from build123d import *

# Parameters (mm, degrees)
SKETCH1_R                = 57.15
SKETCH1_R_2              = 51.1302
SCHEDULED_CHAMBER_DEPTH  = 260.35
SKETCH2_R                = 76.2
SKETCH2_R_2              = 54.102
FLANGE_DEPTH             = 6.35
ORIGINAL_BOLT_HOLE_REACH = 283.771
SKETCH3_R                = 3.175
BOLT_HOLE_PATTERN_COUNT  = 8


with BuildPart() as part:
    # Sketch1 → Scheduled Chamber (new body)
    with BuildSketch(Plane(origin=(0, 0, 0), x_dir=(1, 0, 0), z_dir=(0, 1, 0))):
        with Locations(Location((0, 0, 0), (0, 0, 270))):
            Circle(SKETCH1_R)
        with Locations(Location((0, 0, 0), (0, 0, 270))):
            Circle(SKETCH1_R_2, mode=Mode.SUBTRACT)
    extrude(amount=-SCHEDULED_CHAMBER_DEPTH)

    # Sketch2 → Flange (add)
    with BuildSketch(Plane(origin=(0, 0, 0), x_dir=(1, 0, 0), z_dir=(0, 1, 0))):
        with Locations(Location((0, 0, 0), (0, 0, 270))):
            Circle(SKETCH2_R)
        Circle(SKETCH2_R_2, mode=Mode.SUBTRACT)
    extrude(amount=-FLANGE_DEPTH)

    # Sketch3 → Original Bolt Hole (cut, up to next)
    with BuildSketch(Plane(origin=(0, 0, 0), x_dir=(1, 0, 0), z_dir=(0, 1, 0)), mode=Mode.PRIVATE) as original_bolt_hole_sk1:
        with Locations(Location((0, 68.58, 0), (0, 0, 270))):
            Circle(SKETCH3_R)
    original_bolt_hole_tool1 = extrude(original_bolt_hole_sk1.sketch, amount=-ORIGINAL_BOLT_HOLE_REACH, mode=Mode.PRIVATE) & part.part
    original_bolt_hole = original_bolt_hole_tool1.solids().sort_by_distance((0, 0, -68.58))[0]
    add(original_bolt_hole, mode=Mode.SUBTRACT)

    # Bolt Hole Pattern: Original Bolt Hole ×8 about axis
    bolt_hole_pattern_axis = Axis((0, 0, 0), (0, 1, 0))
    for i in range(1, BOLT_HOLE_PATTERN_COUNT):
        add(original_bolt_hole.rotate(bolt_hole_pattern_axis, i * 360 / BOLT_HOLE_PATTERN_COUNT), mode=Mode.SUBTRACT)


solid = part.part
Can you work these out from the model? Positions are in its coordinate system, mm. A direction names the side the tool comes from. Give positions to 0.01 mm unless a question says otherwise; leave off trailing zeros. Order: outer loops, then holes, each group sorted by start corner. A loop starts at its lowest first (then second) coordinate and runs counter-clockwise, first axis right, second up. Notation, with made-up numbers: (30, -37.5) - (63, -37.5) arc R19 ccw to (63, -30.5) - close; hole circle Ø10 at (29, 66.25). An arc over 180 degrees is marked (long way). Write each question's results on one line, items separated by ' | '.
1) Suppose I cut it at C-C, the plane x = -16. Write out the boundary of the cut face in (y, z).
Final values:
outline: (-260.35, -54.86) - (-6.35, -54.86) - (-6.35, -74.5) - (0, -74.5) - (0, -48.56) - (-260.35, -48.56) - close; (-260.35, 48.56) - (0, 48.56) - (0, 74.5) - (-6.35, 74.5) - (-6.35, 54.86) - (-260.35, 54.86) - close
2) Suppose I cut it at D-D, the plane z = 68.58. Write out the boundary of the cut face in (x, y) (3 decimals).
Final values:
outline: (-33.215, -6.35) - (-3.175, -6.35) - (-3.175, 0) - (-33.215, 0) - close; (3.175, -6.35) - (33.215, -6.35) - (33.215, 0) - (3.175, 0) - close
3) I'm going to push flat-ended pins straight in: pin 1 Ø3 at (x, y) = (-40, -229) entering from +Z; pin 2 Ø12 at (x, z) = (52, -53.5) entering from -Y; pin 3 Ø1 at (x, y) = (-13.5, -105) entering from -Z. Where does each tip first touch, or does it pass through?
Final values:
pin 1: stops at z = 42.24 | pin 2: stops at y = -6.35 | pin 3: stops at z = -55.65
4) Please list where these lines run through material, in increasing order: line 1 along X through (y, z) = (-31, -15); line 2 along Z through (x, y) = (-26, -66.5); line 3 along Y through (x, z) = (27, 52.5). Write a range as [from, to].
Final values:
line 1: x = [-55.15, -48.88], [48.88, 55.15] | line 2: z = [-50.89, -44.03], [44.03, 50.89] | line 3: y = [-6.35, 0]
5) If we mould it in two halves opening along Z, with no side actions, what happens to faces 1 (the face through (-45.678, -3.131, -47.026)), 2 (the face through (2.513, -131.572, -57.095)), 3 (the face through (-29, -260.35, -43))? For each: pulls with the +Z half, pulls with the -Z half, needs draft (parallel to the pull), parting line crosses it, or undercut.
Final values:
face 1: undercut | face 2: parting line crosses it | face 3: needs draft
6) Suppose I cut it at B-B, the plane x = 0. Write out the boundary of the cut face in (y, z) (3 decimals), then the cut area to 3 significant figures.
Final values:
outline: (-260.35, -57.15) - (-6.35, -57.15) - (-6.35, -65.405) - (0, -65.405) - (0, -51.13) - (-260.35, -51.13) - close; (-260.35, 51.13) - (0, 51.13) - (0, 65.405) - (-6.35, 65.405) - (-6.35, 57.15) - (-260.35, 57.15) - close; (-6.35, -76.2) - (0, -76.2) - (0, -71.755) - (-6.35, -71.755) - close; (-6.35, 71.755) - (0, 71.755) - (0, 76.2) - (-6.35, 76.2) - close | area: 3,300 mm^2
7) On a 3-axis mill with a long thin cutter (end or side, diameter ignored), from which of +Z, -Z, +X, -X, +Y, -Y can I reach the whole of each face in a straight line? I mean faces 4 (the face through (51.01, -3.13, -46.56)), 5 (the face through (51, -6.35, -29)). Say none if no direction works.
Final values:
face 4: +Y, -Y | face 5: -Y
8) Suppose I cut it at A-A, the plane z = 0. Write out the boundary of the cut face in (x, y) (3 decimals), then the cut area to 3 significant figures.
Final values:
outline: (-76.2, -6.35) - (-71.755, -6.35) - (-71.755, 0) - (-76.2, 0) - close; (-65.405, -6.35) - (-57.15, -6.35) - (-57.15, -260.35) - (-51.13, -260.35) - (-51.13, 0) - (-65.405, 0) - close; (51.13, -260.35) - (57.15, -260.35) - (57.15, -6.35) - (65.405, -6.35) - (65.405, 0) - (51.13, 0) - close; (71.755, -6.35) - (76.2, -6.35) - (76.2, 0) - (71.755, 0) - close | area: 3,300 mm^2
